Read the model definition and answer for the solid it produces. Units are mm, in the model's axes. Give positions to 0.01 mm unless a question says otherwise; leave off trailing zeros. Order: outer loops, then holes, each group sorted by start corner. A loop starts at its lowest first (then second) coordinate and runs counter-clockwise, first axis right, second up. Notation, with made-up numbers: (19.25, 79.5) - (65.25, 79.5) arc R14 ccw to (65.25, 94.5) - close; hole circle Ø10 at (54.5, -23.75). An arc over 180 degrees is marked (long way). Use a Markdown table: item, result. Add a question column.
1. A cutting plane is placed at A-A on x = 0.55. Determine the outline of the cut face in (y, z).
2. Consider L1, parallel to Y at x = 0.85, z = 5.5; L2, parallel to Y at x = 0.15, z = 48; L3, parallel to Z at x = 0.65, y = -60.5. Determine where each line is inside the solid, lowest interval first.
3. A cutting plane is placed at C-C on z = 59.5. Determine the outline of the cut face in (x, y), and give its area (3 significant figures).
4. A cutting plane is placed at B-B on y = -44. Determine the outline of the cut face in (x, z), and give its area (3 significant figures).
```python
from build123d import *

# Parameters (mm, degrees)
F1_DEPTH = 1


with BuildPart() as f1:
    # F0 (on Right) → F1 (new body)
    with BuildSketch(Plane.YZ):
        with BuildLine():
            Line((-80, 0), (-5, 0))
            ThreePointArc((-5, 0), (-1.464466, 1.464466), (0, 5))
            Line((0, 5), (0, 61.4))
            ThreePointArc((0, 61.4), (-1.464466, 64.935534), (-5, 66.4))
            Line((-5, 66.4), (-40, 66.4))
            ThreePointArc((-40, 66.4), (-69.979813, 39.211936), (-80, 0))
        make_face()
    extrude(amount=F1_DEPTH)


solid = f1.part
```
Output values:
| question | item | result |
|---|---|---|
| 1 | outline | (-80, 0) - (-5, 0) arc R5 ccw to (0, 5) - (0, 61.4) arc R5 ccw to (-5, 66.4) - (-40, 66.4) arc R70.3 ccw to start |
| 2 | L1 | -80.01 to 0 |
| 2 | L2 | -63.72 to 0 |
| 2 | L3 | 0 to 51.6 |
| 3 | outline | (0, -51.51) - (1, -51.51) - (1, 0) - (0, 0) - close |
| 3 | area | 51.5 mm² |
| 4 | outline | (0, 0) - (1, 0) - (1, 64.33) - (0, 64.33) - close |
| 4 | area | 64.3 mm² |
